Geometry check sheet. Reference: the model listing, model coordinates, mm. Give positions to 0.01 mm unless a question says otherwise; leave off trailing zeros. Order: outer loops, then holes, each group sorted by start corner. A loop starts at its lowest first (then second) coordinate and runs counter-clockwise, first axis right, second up. Notation, with made-up numbers: M 77,2 L 87,2 A5 cw 87,7 Z; hole C 79.5,-23.75 d5. An arc over 180 degrees is marked long. Answer as CSV lines item,"result". Start each with the question number.
```python
from build123d import *

# Parameters (mm, degrees)
BOSS_EXTRU_1_DEPTH = 0.225


with BuildPart() as part:
    # Esquisse8 → R_volution2 (revolve)
    with BuildSketch(Plane.XY, mode=Mode.PRIVATE) as r_volution2_sk:
        Polygon((-2.05, 8.55), (-2.5, 8.55), (-2.5, -8.55), (-2.05, -8.55), (0, -8.55), (0, 8.55), align=None)
    revolve(r_volution2_sk.sketch.rotate(Axis((0, 8.55, 0), (0, -1, 0)), 270), axis=Axis((0, 8.55, 0), (0, -1, 0)))

    # Esquisse8_4 → Boss.-Extru.1 (add, symmetric)
    with BuildSketch(Plane.XY):
        with BuildLine():
            Line((-2.05, -8.55), (-2.5, -8.55))
            Line((-2.5, -8.55), (-2.5, -10))
            ThreePointArc((-2.5, -10), (0, -12.5), (2.5, -10))
            Line((2.5, -10), (2.5, -8.55))
            Line((2.5, -8.55), (2.05, -8.55))
            Line((2.05, -8.55), (2.05, -10))
            ThreePointArc((2.05, -10), (0, -12.05), (-2.05, -10))
            Line((-2.05, -10), (-2.05, -8.55))
        make_face()
        with BuildLine():
            ThreePointArc((2.5, 10), (0, 12.5), (-2.5, 10))
            Line((-2.5, 10), (-2.5, 8.55))
            Line((-2.5, 8.55), (-2.05, 8.55))
            Line((-2.05, 8.55), (-2.05, 10))
            ThreePointArc((-2.05, 10), (0, 12.05), (2.05, 10))
            Line((2.05, 10), (2.05, 8.55))
            Line((2.05, 8.55), (2.5, 8.55))
            Line((2.5, 8.55), (2.5, 10))
        make_face()
    extrude(amount=BOSS_EXTRU_1_DEPTH, both=True)


solid = part.part
```
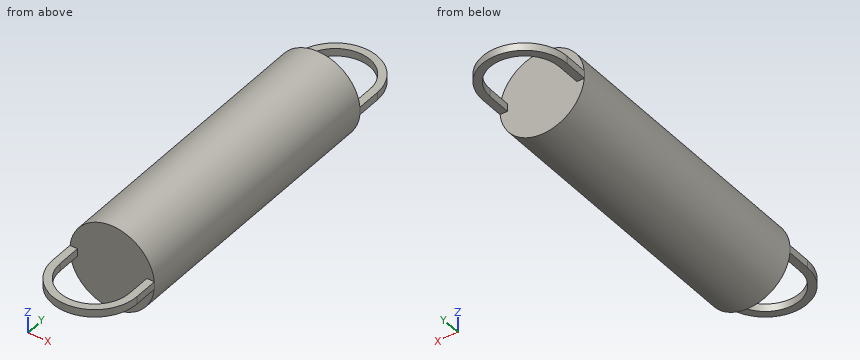
Item 1: Section check B-B on y = -9.75. Record the boundary of the cut face in (x, z) (3 decimals), then the cut area to 3 significant figures.
Item 2: Section check D-D on x = 1.1. Record the boundary of the cut face in (y, z) (3 decimals), then the cut area to 3 significant figures.
Item 3: Section check C-C on z = 0.7. Record the boundary of the cut face in (x, y), then the cut area to 3 significant figures.
Item 4: Section check A-A on x = 0. Record the boundary of the cut face in (y, z) (3 decimals), then the cut area to 3 significant figures.
Item 5: Depth check by flat-ended pin: pin 1 Ø1 at (x, z) = (-1, 0) entering from +Y; pin 2 Ø2 at (y, z) = (-10, 0.5) entering from -X; pin 3 Ø1.5 at (x, z) = (-2, 1.5) entering from +Y; pin 4 Ø3 at (x, y) = (-1, 11) entering from -Z (3 decimals). Enter the tip coordinate at first touch or a pass-through.
Item 6: Scan lines: line 1 along Y through (x, z) = (-0.15, -0.6); line 2 along Y through (x, z) = (-1.65, 0); line 3 along Z through (x, y) = (2.15, -9) (3 decimals). Record each from-to range of solid material in increasing order.
Numbers:
1,outline,"M -2.5,-0.225 L -2.05,-0.225 L -2.05,0.225 L -2.5,0.225 Z; M 2.05,-0.225 L 2.5,-0.225 L 2.5,0.225 L 2.05,0.225 Z"
1,area,"0.405 mm2"
2,outline,"M -12.245,-0.225 L -11.73,-0.225 L -11.73,0.225 L -12.245,0.225 Z; M -8.55,-2.245 L 8.55,-2.245 L 8.55,2.245 L -8.55,2.245 Z; M 11.73,-0.225 L 12.245,-0.225 L 12.245,0.225 L 11.73,0.225 Z"
2,area,"77.2 mm2"
3,outline,"M -2.4,-8.55 L 2.4,-8.55 L 2.4,8.55 L -2.4,8.55 Z"
3,area,"82.1 mm2"
4,outline,"M -12.5,-0.225 L -12.05,-0.225 L -12.05,0.225 L -12.5,0.225 Z; M -8.55,-2.5 L 8.55,-2.5 L 8.55,2.5 L -8.55,2.5 Z; M 12.05,-0.225 L 12.5,-0.225 L 12.5,0.225 L 12.05,0.225 Z"
4,area,"85.9 mm2"
5,pin 1,"y = 12.45"
5,pin 2,"x = -2.5"
5,pin 3,"y = 8.55"
5,pin 4,"z = -0.225"
6,line 1,"-8.55 to 8.55"
6,line 2,"-11.88 to -11.22, -8.55 to 8.55, 11.22 to 11.88"
6,line 3,"-0.225 to 0.225"
